Can you work these out from the model? Positions are in its coordinate system, mm. Face numbers are marked on the shaded views. A direction names the side the tool comes from. Coordinates: 2 decimals unless noted, no trailing zeros. Loops run counter-clockwise (first coordinate to the right, second up) from the corner with the lowest first, then second, coordinate; pieces in that order, holes last.
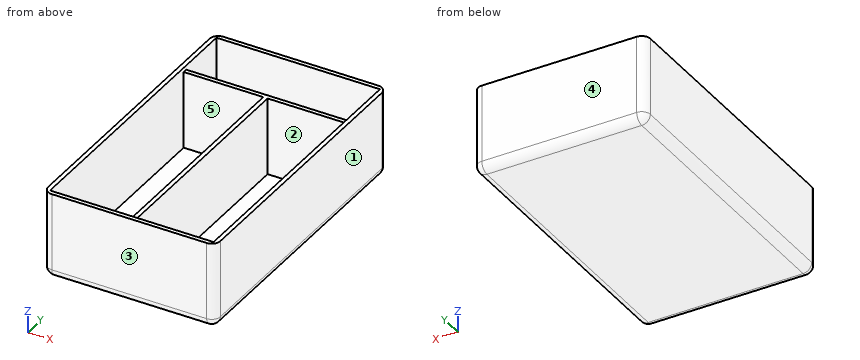
```python
from build123d import *

# Parameters (mm, degrees)
F0_W     = 100
F0_H     = 170
F1_DEPTH = 50
F2_T     = -2.5
F3_R     = 5
F4_W     = 95
F4_H     = 2.5
F5_DEPTH = 45
F6_W     = 2.5
F6_H     = 132.5
F7_DEPTH = 45


with BuildPart() as f1:
    # F0 (on Top) → F1 (new body)
    with BuildSketch(Plane.XY):
        with Locations((50, 85)):
            Rectangle(F0_W, F0_H)
    extrude(amount=F1_DEPTH)

    # F2
    f2_openings = [f1.faces().sort_by_distance(p)[0] for p in [
        (50, 85, 50),
    ]]
    offset(amount=F2_T, openings=f2_openings)

    # F3
    f3_edges = [f1.edges().sort_by_distance(p)[0] for p in [
        (100, 170, 25),
        (100, 85, 0),
        (100, 0, 25),
        (0, 0, 25),
        (50, 0, 0),
        (0, 85, 0),
        (50, 170, 0),
        (0, 170, 25),
    ]]
    fillet(f3_edges, radius=F3_R)

    # F4 (on face) → F5 (join)
    with BuildSketch(Plane.XY.offset(2.5)):
        with Locations((50, 136.25)):
            Rectangle(F4_W, F4_H)
    extrude(amount=F5_DEPTH)

    # F6 (on face) → F7 (join)
    with BuildSketch(Plane.XY.offset(2.5)):
        with Locations((50, 68.75)):
            Rectangle(F6_W, F6_H)
    extrude(amount=F7_DEPTH)


solid = f1.part
```
Item 1: On a 3-axis mill with a long thin cutter (end or side, diameter ignored), from which of +Z, -Z, +X, -X, +Y, -Y can I reach the whole of each face in a straight line? I mean the marked faces 4 and 5. Say none if no direction works.
Results are:
face 4: +Z, -Z, +X, -X, +Y
face 5: +Z
Item 2: Suppose I cut it at B-B, the plane y = 47.5. Please give me the cut outline in (x, z).
Results are:
outline: (0, 5) arc R5 ccw to (5, 0) - (95, 0) arc R5 ccw to (100, 5) - (100, 50) - (97.5, 50) - (97.5, 2.5) - (51.25, 2.5) - (51.25, 47.5) - (48.75, 47.5) - (48.75, 2.5) - (2.5, 2.5) - (2.5, 50) - (0, 50) - close
Item 3: We'd pull the mould along Y, two halves only. Please class the marked faces 1, 2 and 3: +Y half, -Y half, draft (parallel to the pull), parting line (faces both ways), or undercut.
Results are:
face 1: draft
face 2: undercut
face 3: -Y half
Item 4: Suppose I cut it at C-C, the plane x = 53. Please give me the cut outline in (y, z).
Results are:
outline: (0, 5) arc R5 ccw to (5, 0) - (165, 0) arc R5 ccw to (170, 5) - (170, 50) - (167.5, 50) - (167.5, 2.5) - (137.5, 2.5) - (137.5, 47.5) - (135, 47.5) - (135, 2.5) - (2.5, 2.5) - (2.5, 50) - (0, 50) - close
Item 5: Suppose I cut it at A-A, the plane z = 7. Please give me the cut outline in (x, y), plus the area to 3 significant figures.
Results are:
outline: (0, 5) arc R5 ccw to (5, 0) - (95, 0) arc R5 ccw to (100, 5) - (100, 165) arc R5 ccw to (95, 170) - (5, 170) arc R5 ccw to (0, 165) - close; hole (2.5, 2.5) - (48.75, 2.5) - (48.75, 135) - (2.5, 135) - close; hole (2.5, 137.5) - (97.5, 137.5) - (97.5, 167.5) - (2.5, 167.5) - close; hole (51.25, 2.5) - (97.5, 2.5) - (97.5, 135) - (51.25, 135) - close
area: 1,870 mm2
Item 6: I'm going to push a flat-ended pin straight in: P1, Ø10, axis at x = 42.5, y = 19.5, coming from the +Z side. Where does the tip first touch, or does it pass through?
Results are:
P1: stops at z = 2.5
Item 7: I need wall thicknesses on line 1 along Y through (x, z) = (48.5, 5); line 2 along X through (y, z) = (44, 40); line 3 along Z through (x, y) = (8, 88). Which ranges of each line are inside material? Lowest first, please.
Results are:
line 1: y = 0 to 2.5, 135 to 137.5, 167.5 to 170
line 2: x = 0 to 2.5, 48.75 to 51.25, 97.5 to 100
line 3: z = 0 to 2.5
